Model file for the job. Use its own axes, mm. Face numbers are marked on the shaded views. Coordinates: 2 decimals unless noted, no trailing zeros. Order: outer loops, then holes, each group sorted by start corner. A loop starts at its lowest first (then second) coordinate and runs counter-clockwise, first axis right, second up.
from build123d import *

# Parameters (mm, degrees)
EXTRUDE1_DEPTH                   = 16
F_1_4_CLEARANCE_HOLE1_AT_2_COUNT = 2
F_1_4_CLEARANCE_HOLE1_AT_2_PITCH = 25.4
F_1_4_CLEARANCE_HOLE1_AT_3_COUNT = 2
F_1_4_CLEARANCE_HOLE1_AT_3_PITCH = 25.4


with BuildPart() as part:
    # Sketch1 → Extrude1 (new body)
    with BuildSketch(Plane(origin=(0, 0, 0), x_dir=(1, 0, 0), z_dir=(0, 1, 0))):
        with BuildLine():
            Line((-25.4, 12.7), (25.4, 12.7))
            ThreePointArc((25.4, 12.7), (38.1, 0), (25.4, -12.7))
            Line((25.4, -12.7), (-25.4, -12.7))
            ThreePointArc((-25.4, -12.7), (-38.1, 0), (-25.4, 12.7))
        make_face()
    extrude(amount=-EXTRUDE1_DEPTH)

    # Sketch2 → 1/4 Clearance Hole1 (revolve, cut)
    with BuildSketch(Plane(origin=(0, 0, 0), x_dir=(0, 0, 1), z_dir=(1, 0, 0))):
        Polygon((0, 0), (0, 16), (3.8989, 16), (3.2639, 15.365), (3.2639, 0.635), (3.8989, 0), align=None)
    f_1_4_clearance_hole1 = revolve(axis=Axis((0, 6.35, 0), (0, -1, 0)), mode=Mode.SUBTRACT)

    # 1/4 Clearance Hole1 at 2: 1/4 Clearance Hole1 ×2
    with Locations(*[(-i * F_1_4_CLEARANCE_HOLE1_AT_2_PITCH, 0, 0) for i in range(1, F_1_4_CLEARANCE_HOLE1_AT_2_COUNT)]):
        add(f_1_4_clearance_hole1, mode=Mode.SUBTRACT)

    # 1/4 Clearance Hole1 at 3: 1/4 Clearance Hole1 ×2
    with Locations(*[(i * F_1_4_CLEARANCE_HOLE1_AT_3_PITCH, 0, 0) for i in range(1, F_1_4_CLEARANCE_HOLE1_AT_3_COUNT)]):
        add(f_1_4_clearance_hole1, mode=Mode.SUBTRACT)


solid = part.part
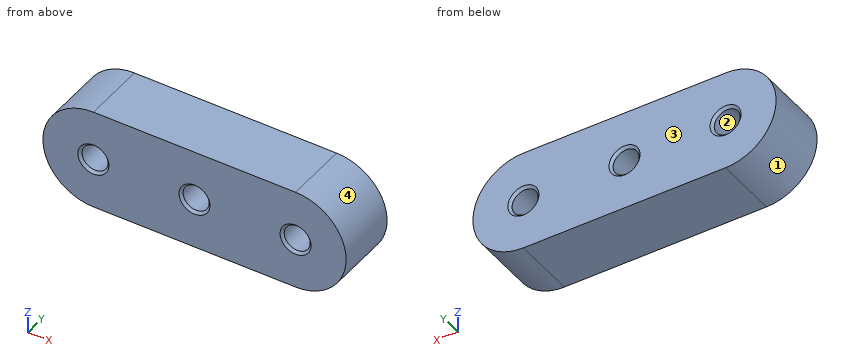
Q1. Cut at A-A, the plane y = -1.5. List the corners of the cut face in (x, z).
Established:
outline: (-25.4, -12.7) - (25.4, -12.7) arc R12.7 ccw to (25.4, 12.7) - (-25.4, 12.7) arc R12.7 ccw to start; hole circle Ø6.53 at (-25.4, 0); hole circle Ø6.53 at (0, 0); hole circle Ø6.53 at (25.4, 0)
Q2. Cut at B-B, the plane x = 0. List the corners of the cut face in (y, z) (3 decimals), plus the area to 3 significant figures.
Established:
outline: (-16, -12.7) - (0, -12.7) - (0, -3.899) - (-0.635, -3.264) - (-15.365, -3.264) - (-16, -3.899) - close; (-16, 3.899) - (-15.365, 3.264) - (-0.635, 3.264) - (0, 3.899) - (0, 12.7) - (-16, 12.7) - close
area: 301 mm2
Q3. Mould opens along X. For the marked faces 1, 2, 3 and 4 say: pulls with the +X half, pulls with the -X half, needs draft (parallel to the pull), parting line crosses it, or undercut.
Established:
face 1: pulls with the -X half
face 2: undercut
face 3: needs draft
face 4: pulls with the +X half
Q4. Drop flat-ended pins along their axis: P1, Ø5, axis at y = -6, z = -8, coming from the +X side; P2, Ø1, axis at y = -11, z = -4.5, coming from the -X side. Give the stop position or say it passes through.
Established:
P1: stops at x = 36.85
P2: stops at x = -37.45
Q5. Cut at D-D, the plane z = -7. List the corners of the cut face in (x, y).
Established:
outline: (-36, -16) - (36, -16) - (36, 0) - (-36, 0) - close
Q6. Cut at C-C, the plane z = 0. List the corners of the cut face in (x, y) (3 decimals).
Established:
outline: (-38.1, -16) - (-29.299, -16) - (-28.664, -15.365) - (-28.664, -0.635) - (-29.299, 0) - (-38.1, 0) - close; (-22.136, -15.365) - (-21.501, -16) - (-3.899, -16) - (-3.264, -15.365) - (-3.264, -0.635) - (-3.899, 0) - (-21.501, 0) - (-22.136, -0.635) - close; (3.264, -15.365) - (3.899, -16) - (21.501, -16) - (22.136, -15.365) - (22.136, -0.635) - (21.501, 0) - (3.899, 0) - (3.264, -0.635) - close; (28.664, -15.365) - (29.299, -16) - (38.1, -16) - (38.1, 0) - (29.299, 0) - (28.664, -0.635) - close
Q7. Probe line 1 (X direction, y = -9.5, z = 0); line 2 (Z direction, x = -25.4, y = -6); line 3 (X direction, y = -11.25, z = -2.5). List the from-to ranges inside material, lowest first.
Established:
line 1: x = -38.1 to -28.66, -22.14 to -3.26, 3.26 to 22.14, 28.66 to 38.1
line 2: z = -12.7 to -3.26, 3.26 to 12.7
line 3: x = -37.85 to -27.5, -23.3 to -2.1, 2.1 to 23.3, 27.5 to 37.85
